Here's how the part is built. I have some questions about the finished solid (model axes, mm). Round coordinates to 2 decimals unless told otherwise and drop trailing zeros. Order: outer loops, then holes, each group sorted by start corner. A loop starts at its lowest first (then second) coordinate and runs counter-clockwise, first axis right, second up. Notation, with made-up numbers: (-33, 36) -> (-16, 36) arc R10 ccw to (-16, 48) -> close; hole circle Ø7 at (58, 47.25). An arc over 180 degrees is marked (long way). Use a Markdown table: item, result. Add a question column.
from build123d import *

# Parameters (mm, degrees)
CROQUIS1_R              = 8.5
CROQUIS1_R_2            = 3
SALIENTE_EXTRUIR1_DEPTH = 6


with BuildPart() as part:
    # Croquis1 → Saliente-Extruir1 (new body)
    with BuildSketch(Plane(origin=(0, 0, 0), x_dir=(1, 0, 0), z_dir=(0, 1, 0))):
        with BuildLine():
            Line((-9.210109587, -6.014472661), (-19.641820946, 9.959862948))
            ThreePointArc((-19.641820946, 9.959862948), (-19.860537089, 15.059054149), (-15.489180854, 17.693600092))
            Line((-15.489180854, 17.693600092), (-1.471942871, 17.788284087))
            Line((-1.471942871, 17.788284087), (11.737098306, 20.363042988))
            ThreePointArc((11.737098306, 20.363042988), (16.549311947, 18.638859347), (17.33162249, 13.587305173))
            Line((17.33162249, 13.587305173), (10.203398333, -4.109825113))
            ThreePointArc((10.203398333, -4.109825113), (1.074046649, -10.947439143), (-9.210109587, -6.014472661))
        make_face()
        with Locations(Location((0, 0, 0), (0, 0, 270))):
            Circle(CROQUIS1_R, mode=Mode.SUBTRACT)
        with Locations(Location((-15.455407497, 12.693714157, 0), (0, 0, 270))):
            Circle(CROQUIS1_R_2, mode=Mode.SUBTRACT)
        with Locations(Location((12.693714157, 15.455407497, 0), (0, 0, 270))):
            Circle(CROQUIS1_R_2, mode=Mode.SUBTRACT)
    extrude(amount=SALIENTE_EXTRUIR1_DEPTH)


solid = part.part
(1) Please list where these lines run through material, in increasing order: probe 1 along X at (y, z) = (1.05, -12); probe 2 along Z at (x, y) = (4, 3.25); probe 3 along X at (y, z) = (1.5, 0). Write a range as from..to.
(2) If we mould it in two halves opening along X, with no side actions, what happens to faces 1 (the cylindrical face through (-18.117, 2.958, -11.309)), 2 (the flat face through (3.1, 0, -8.4)), 3 (the flat face through (5.04, 2.958, -19.058))? For each: pulls with the +X half, pulls with the -X half, needs draft (parallel to the pull), parting line crosses it, or undercut.
(3) I want a section at B-B on y = 1.6. List the corners of the cut face in (x, z) for me.
(4) I want a section at A-A on x = -6. List the corners of the cut face in (y, z) for me.
(5) I want a section at D-D on x = -10.5. List the corners of the cut face in (y, z) for me, and give its area (3 significant figures).
(6) I want a section at C-C on z = 0. List the corners of the cut face in (x, y) for me, and give its area (3 significant figures).
(7) I'm going to push flat-ended pins straight in: P1, Ø1.5, axis at y = 2.5, z = 1, coming from the +X side; P2, Ø15.5, axis at x = 0, z = 0, coming from the +Y side; P3, Ø5, axis at x = -10, z = 7.5, coming from the -Y side; P4, Ø1, axis at x = -6, y = 4.5, coming from the -Z side. Where does each tip first touch, or does it pass through?
Output:
| question | item | result |
|---|---|---|
| 1 | probe 1 | -20.41..-18.37, -12.54..16.69 |
| 1 | probe 2 | -18.85..-7.5, 7.5..10.25 |
| 1 | probe 3 | -13.14..-8.5, 8.5..11.86 |
| 2 | face 1 | undercut |
| 2 | face 2 | needs draft |
| 2 | face 3 | pulls with the -X half |
| 3 | outline | (-19.64, -9.96) arc R5 ccw to (-15.49, -17.69) -> (-1.47, -17.79) -> (11.74, -20.36) arc R5 ccw to (17.33, -13.59) -> (10.2, 4.11) arc R11 ccw to (-9.21, 6.01) -> close; hole circle Ø6 at (-15.46, -12.69); hole circle Ø17 at (0, 0); hole circle Ø6 at (12.69, -15.46) |
| 4 | outline | (0, -17.76) -> (6, -17.76) -> (6, -6.02) -> (0, -6.02) -> close; (0, 6.02) -> (6, 6.02) -> (6, 9.22) -> (0, 9.22) -> close |
| 5 | outline | (0, -17.73) -> (6, -17.73) -> (6, 4.04) -> (0, 4.04) -> close |
| 5 | area | 131 mm² |
| 6 | outline | (-13.14, 0) -> (-8.5, 0) -> (-8.5, 6) -> (-13.14, 6) -> close; (8.5, 0) -> (11.86, 0) -> (11.86, 6) -> (8.5, 6) -> close |
| 6 | area | 48.0 mm² |
| 7 | P1 | x = 11.76 |
| 7 | P2 | through |
| 7 | P3 | y = 0 |
| 7 | P4 | z = -17.76 |
